Geometry: final body of the model. Coordinates: model frame, mm. Face numbers are marked on the shaded views. A direction names the side the tool comes from. Round coordinates to 2 decimals unless told otherwise and drop trailing zeros. Loops run counter-clockwise (first coordinate to the right, second up) from the corner with the lowest first, then second, coordinate; pieces in that order, holes last. Notation, with made-up numbers: (86.25, -8.75) -> (108.25, -8.75) arc R20 ccw to (108.25, 4.25) -> close; hole circle Ø3 at (85.5, 6). An arc over 180 degrees is marked (long way). Answer in a Markdown table with one row per item.
```python
from build123d import *

# Parameters (mm, degrees)
EXTRUDE_1_DEPTH     = 200
CUT_EXTRUDE_1_DEPTH = 195
CUT_EXTRUDE_4_REACH = 443.251
SKETCH_9_R          = 9
CUT_EXTRUDE_5_REACH = 344.504
SKETCH_11_R         = 1.6
CUT_EXTRUDE_6_REACH = 344.504
SKETCH_12_R         = 1.6
CUT_EXTRUDE_7_REACH = 344.504
SKETCH_13_R         = 2.5
SKETCH_14_W         = 5
SKETCH_14_H         = 193
EXTRUDE_2_DEPTH     = 195
CUT_EXTRUDE_8_REACH = 344.504
SKETCH_15_R         = 2
SKETCH_15_R_2       = 9
CUT_EXTRUDE_9_REACH = 297.565
SKETCH_16_R         = 9


with BuildPart() as part:
    # 草图1 → 凸台-拉伸1 (new body)
    with BuildSketch(Plane(origin=(0, 0, 0), x_dir=(1, 0, 0), z_dir=(0, 1, 0))):
        Polygon((-190, 78.5), (-190, 101.5), (-167, 101.5), (167, 101.5), (190, 101.5), (190, 78.5), (190, -78.5), (190, -101.5), (167, -101.5), (-167, -101.5), (-190, -101.5), (-190, -78.5), align=None)
    extrude(amount=EXTRUDE_1_DEPTH)

    # 草图3 → 切除-拉伸1 (cut)
    with BuildSketch(Plane(origin=(0, 200, 0), x_dir=(1, 0, 0), z_dir=(0, 1, 0))):
        Polygon((-167, 96.5), (167, 96.5), (185, 96.5), (185, 78.5), (185, -78.5), (185, -96.5), (167, -96.5), (-167, -96.5), (-185, -96.5), (-185, -78.5), (-185, 78.5), (-185, 96.5), align=None)
    extrude(amount=-CUT_EXTRUDE_1_DEPTH, mode=Mode.SUBTRACT)

    # 草图9 → 切除-拉伸4 (cut, up to next)
    with BuildSketch(Plane(origin=(190, 0, 0), x_dir=(0, 0, -1), z_dir=(1, 0, 0)), mode=Mode.PRIVATE) as cut_extrude_4_sk1:
        with Locations((53.5, 170)):
            Circle(SKETCH_9_R)
    cut_extrude_4_tool1 = extrude(cut_extrude_4_sk1.sketch, amount=-CUT_EXTRUDE_4_REACH, mode=Mode.PRIVATE) & part.part
    add(cut_extrude_4_tool1.solids().sort_by_distance((190, 170, -53.5))[0], mode=Mode.SUBTRACT)

    # 草图11 → 切除-拉伸5 (cut, up to next)
    with BuildSketch(Plane.XY.offset(101.5), mode=Mode.PRIVATE) as cut_extrude_5_sk1:
        with Locations((77, 180)):
            Circle(SKETCH_11_R)
    cut_extrude_5_tool1 = extrude(cut_extrude_5_sk1.sketch, amount=-CUT_EXTRUDE_5_REACH, mode=Mode.PRIVATE) & part.part
    # 草图11 → 切除-拉伸5 (cut, up to next)
    with BuildSketch(Plane.XY.offset(101.5), mode=Mode.PRIVATE) as cut_extrude_5_sk2:
        with Locations((147, 180)):
            Circle(SKETCH_11_R)
    cut_extrude_5_tool2 = extrude(cut_extrude_5_sk2.sketch, amount=-CUT_EXTRUDE_5_REACH, mode=Mode.PRIVATE) & part.part
    # 草图11 → 切除-拉伸5 (cut, up to next)
    with BuildSketch(Plane.XY.offset(101.5), mode=Mode.PRIVATE) as cut_extrude_5_sk3:
        with Locations((77, 110)):
            Circle(SKETCH_11_R)
    cut_extrude_5_tool3 = extrude(cut_extrude_5_sk3.sketch, amount=-CUT_EXTRUDE_5_REACH, mode=Mode.PRIVATE) & part.part
    # 草图11 → 切除-拉伸5 (cut, up to next)
    with BuildSketch(Plane.XY.offset(101.5), mode=Mode.PRIVATE) as cut_extrude_5_sk4:
        with Locations((147, 110)):
            Circle(SKETCH_11_R)
    cut_extrude_5_tool4 = extrude(cut_extrude_5_sk4.sketch, amount=-CUT_EXTRUDE_5_REACH, mode=Mode.PRIVATE) & part.part
    add(cut_extrude_5_tool1.solids().sort_by_distance((77, 180, 101.5))[0], mode=Mode.SUBTRACT)
    add(cut_extrude_5_tool2.solids().sort_by_distance((147, 180, 101.5))[0], mode=Mode.SUBTRACT)
    add(cut_extrude_5_tool3.solids().sort_by_distance((77, 110, 101.5))[0], mode=Mode.SUBTRACT)
    add(cut_extrude_5_tool4.solids().sort_by_distance((147, 110, 101.5))[0], mode=Mode.SUBTRACT)

    # 草图12 → 切除-拉伸6 (cut, up to next)
    with BuildSketch(Plane.XY.offset(101.5), mode=Mode.PRIVATE) as cut_extrude_6_sk1:
        with Locations((77, 145)):
            Circle(SKETCH_12_R)
    cut_extrude_6_tool1 = extrude(cut_extrude_6_sk1.sketch, amount=-CUT_EXTRUDE_6_REACH, mode=Mode.PRIVATE) & part.part
    # 草图12 → 切除-拉伸6 (cut, up to next)
    with BuildSketch(Plane.XY.offset(101.5), mode=Mode.PRIVATE) as cut_extrude_6_sk2:
        with Locations((112.496378105, 179.496480131)):
            Circle(SKETCH_12_R)
    cut_extrude_6_tool2 = extrude(cut_extrude_6_sk2.sketch, amount=-CUT_EXTRUDE_6_REACH, mode=Mode.PRIVATE) & part.part
    # 草图12 → 切除-拉伸6 (cut, up to next)
    with BuildSketch(Plane.XY.offset(101.5), mode=Mode.PRIVATE) as cut_extrude_6_sk3:
        with Locations((146.992858236, 144.000102025)):
            Circle(SKETCH_12_R)
    cut_extrude_6_tool3 = extrude(cut_extrude_6_sk3.sketch, amount=-CUT_EXTRUDE_6_REACH, mode=Mode.PRIVATE) & part.part
    # 草图12 → 切除-拉伸6 (cut, up to next)
    with BuildSketch(Plane.XY.offset(101.5), mode=Mode.PRIVATE) as cut_extrude_6_sk4:
        with Locations((111.496480131, 109.503621895)):
            Circle(SKETCH_12_R)
    cut_extrude_6_tool4 = extrude(cut_extrude_6_sk4.sketch, amount=-CUT_EXTRUDE_6_REACH, mode=Mode.PRIVATE) & part.part
    add(cut_extrude_6_tool1.solids().sort_by_distance((77, 145, 101.5))[0], mode=Mode.SUBTRACT)
    add(cut_extrude_6_tool2.solids().sort_by_distance((112.496378, 179.49648, 101.5))[0], mode=Mode.SUBTRACT)
    add(cut_extrude_6_tool3.solids().sort_by_distance((146.992858, 144.000102, 101.5))[0], mode=Mode.SUBTRACT)
    add(cut_extrude_6_tool4.solids().sort_by_distance((111.49648, 109.503622, 101.5))[0], mode=Mode.SUBTRACT)

    # 草图13 → 切除-拉伸7 (cut, up to next)
    with BuildSketch(Plane.XY.offset(101.5), mode=Mode.PRIVATE) as cut_extrude_7_sk1:
        with Locations((99, 42.5)):
            Circle(SKETCH_13_R)
    cut_extrude_7_tool1 = extrude(cut_extrude_7_sk1.sketch, amount=-CUT_EXTRUDE_7_REACH, mode=Mode.PRIVATE) & part.part
    # 草图13 → 切除-拉伸7 (cut, up to next)
    with BuildSketch(Plane.XY.offset(101.5), mode=Mode.PRIVATE) as cut_extrude_7_sk2:
        with Locations((151, 42.5)):
            Circle(SKETCH_13_R)
    cut_extrude_7_tool2 = extrude(cut_extrude_7_sk2.sketch, amount=-CUT_EXTRUDE_7_REACH, mode=Mode.PRIVATE) & part.part
    add(cut_extrude_7_tool1.solids().sort_by_distance((99, 42.5, 101.5))[0], mode=Mode.SUBTRACT)
    add(cut_extrude_7_tool2.solids().sort_by_distance((151, 42.5, 101.5))[0], mode=Mode.SUBTRACT)

    # 草图14 → 凸台-拉伸2 (add)
    with BuildSketch(Plane(origin=(0, 5, 0), x_dir=(1, 0, 0), z_dir=(0, 1, 0))):
        Rectangle(SKETCH_14_W, SKETCH_14_H)
    extrude(amount=EXTRUDE_2_DEPTH)

    # 草图15 → 切除-拉伸8 (cut, up to next)
    with BuildSketch(Plane(origin=(0, 0, -101.5), x_dir=(-1, 0, 0), z_dir=(0, 0, -1)), mode=Mode.PRIVATE) as cut_extrude_8_sk1:
        with Locations((-155, 120)):
            Circle(SKETCH_15_R)
    cut_extrude_8_tool1 = extrude(cut_extrude_8_sk1.sketch, amount=-CUT_EXTRUDE_8_REACH, mode=Mode.PRIVATE) & part.part
    # 草图15 → 切除-拉伸8 (cut, up to next)
    with BuildSketch(Plane(origin=(0, 0, -101.5), x_dir=(-1, 0, 0), z_dir=(0, 0, -1)), mode=Mode.PRIVATE) as cut_extrude_8_sk2:
        with Locations((-78.5, 120)):
            Circle(SKETCH_15_R)
    cut_extrude_8_tool2 = extrude(cut_extrude_8_sk2.sketch, amount=-CUT_EXTRUDE_8_REACH, mode=Mode.PRIVATE) & part.part
    # 草图15 → 切除-拉伸8 (cut, up to next)
    with BuildSketch(Plane(origin=(0, 0, -101.5), x_dir=(-1, 0, 0), z_dir=(0, 0, -1)), mode=Mode.PRIVATE) as cut_extrude_8_sk3:
        with Locations((-78.5, 65)):
            Circle(SKETCH_15_R)
    cut_extrude_8_tool3 = extrude(cut_extrude_8_sk3.sketch, amount=-CUT_EXTRUDE_8_REACH, mode=Mode.PRIVATE) & part.part
    # 草图15 → 切除-拉伸8 (cut, up to next)
    with BuildSketch(Plane(origin=(0, 0, -101.5), x_dir=(-1, 0, 0), z_dir=(0, 0, -1)), mode=Mode.PRIVATE) as cut_extrude_8_sk4:
        with Locations((-155, 65)):
            Circle(SKETCH_15_R)
    cut_extrude_8_tool4 = extrude(cut_extrude_8_sk4.sketch, amount=-CUT_EXTRUDE_8_REACH, mode=Mode.PRIVATE) & part.part
    # 草图15 → 切除-拉伸8 (cut, up to next)
    with BuildSketch(Plane(origin=(0, 0, -101.5), x_dir=(-1, 0, 0), z_dir=(0, 0, -1)), mode=Mode.PRIVATE) as cut_extrude_8_sk5:
        with Locations((-25, 170)):
            Circle(SKETCH_15_R_2)
    cut_extrude_8_tool5 = extrude(cut_extrude_8_sk5.sketch, amount=-CUT_EXTRUDE_8_REACH, mode=Mode.PRIVATE) & part.part
    add(cut_extrude_8_tool1.solids().sort_by_distance((155, 120, -101.5))[0], mode=Mode.SUBTRACT)
    add(cut_extrude_8_tool2.solids().sort_by_distance((78.5, 120, -101.5))[0], mode=Mode.SUBTRACT)
    add(cut_extrude_8_tool3.solids().sort_by_distance((78.5, 65, -101.5))[0], mode=Mode.SUBTRACT)
    add(cut_extrude_8_tool4.solids().sort_by_distance((155, 65, -101.5))[0], mode=Mode.SUBTRACT)
    add(cut_extrude_8_tool5.solids().sort_by_distance((25, 170, -101.5))[0], mode=Mode.SUBTRACT)

    # 草图16 → 切除-拉伸9 (cut, up to next)
    with BuildSketch(Plane(origin=(2.5, 0, 0), x_dir=(0, 0, -1), z_dir=(1, 0, 0)), mode=Mode.PRIVATE) as cut_extrude_9_sk1:
        with Locations((53.5, 170)):
            Circle(SKETCH_16_R)
    cut_extrude_9_tool1 = extrude(cut_extrude_9_sk1.sketch, amount=-CUT_EXTRUDE_9_REACH, mode=Mode.PRIVATE) & part.part
    add(cut_extrude_9_tool1.solids().sort_by_distance((2.5, 170, -53.5))[0], mode=Mode.SUBTRACT)


solid = part.part
```
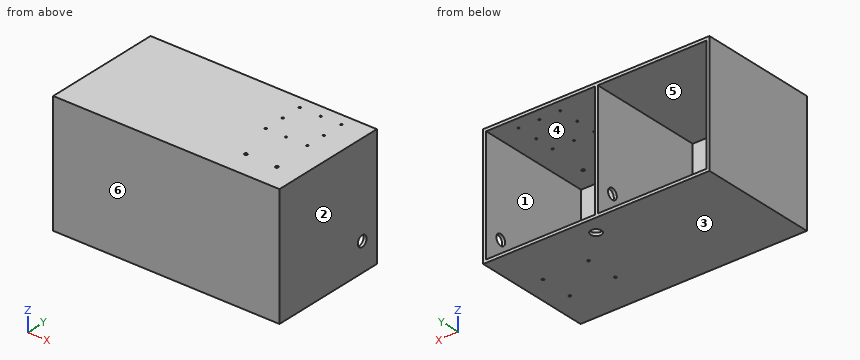
Item 1: Section query A-A, the plane y = 170. Output: boundary loops of the cut face in (x, z), and give its area (4 significant figures).
Ans:
| item | result |
|---|---|
| outline | (-190, -101.5) -> (16, -101.5) -> (16, -96.5) -> (2.5, -96.5) -> (2.5, -62.5) -> (-2.5, -62.5) -> (-2.5, -96.5) -> (-185, -96.5) -> (-185, 96.5) -> (-2.5, 96.5) -> (-2.5, -44.5) -> (2.5, -44.5) -> (2.5, 96.5) -> (185, 96.5) -> (185, -44.5) -> (190, -44.5) -> (190, 101.5) -> (-190, 101.5) -> close; (34, -101.5) -> (190, -101.5) -> (190, -62.5) -> (185, -62.5) -> (185, -96.5) -> (34, -96.5) -> close |
| area | 6,425 mm2 |
Item 2: Ray query, L1, parallel to Y at x = 147, z = 98; L2, parallel to X at y = 88, z = 2; L3, parallel to Y at x = 77, z = 98. Return the intervals inside material, ascending.
Ans:
| item | result |
|---|---|
| L1 | 0 to 108.4, 111.6 to 142.4, 145.6 to 178.4, 181.6 to 200 |
| L2 | -190 to -185, -2.5 to 2.5, 185 to 190 |
| L3 | 0 to 108.4, 111.6 to 143.4, 146.6 to 178.4, 181.6 to 200 |
Item 3: Section query B-B, the plane x = 121. Output: boundary loops of the cut face in (y, z), and give its area (4 significant figures).
Ans:
| item | result |
|---|---|
| outline | (0, -101.5) -> (200, -101.5) -> (200, -96.5) -> (5, -96.5) -> (5, 96.5) -> (200, 96.5) -> (200, 101.5) -> (0, 101.5) -> close |
| area | 2,965 mm2 |
Item 4: Section query C-C, the plane z = -77. Output: boundary loops of the cut face in (x, y), and give its area (4 significant figures).
Ans:
| item | result |
|---|---|
| outline | (-190, 0) -> (190, 0) -> (190, 200) -> (185, 200) -> (185, 5) -> (2.5, 5) -> (2.5, 200) -> (-2.5, 200) -> (-2.5, 5) -> (-185, 5) -> (-185, 200) -> (-190, 200) -> close |
| area | 4,825 mm2 |
Item 5: First-contact query: P1, Ø1.9, axis at x = 146.99, y = 144, coming from the +Z side. Flat tip, straight axial feed; report the tip coordinate or a pass-through.
Ans:
| item | result |
|---|---|
| P1 | z = -96.5 |
Item 6: Mould query, pull axis X, two halves, no side actions, for the marked faces 1, 2, 3 and 4. Classes: released by +X, released by -X, zero draft, split by the parting line, or undercut.
Ans:
| item | result |
|---|---|
| face 1 | undercut |
| face 2 | released by +X |
| face 3 | zero draft |
| face 4 | undercut |
Item 7: Set-up query: the marked faces 5 and 6. Return all of +Z, -Z, +X, -X, +Y, -Y with unobstructed straight access to the full face (end or side cutting, diameter ignored); none if empty.
Ans:
| item | result |
|---|---|
| face 5 | +Y |
| face 6 | +Z, -Z, +X, -X, -Y |
